Geometry check sheet. Reference: the model listing, model coordinates, mm. A direction names the side the tool comes from. Round coordinates to 2 decimals unless told otherwise and drop trailing zeros. Loops run counter-clockwise (first coordinate to the right, second up) from the corner with the lowest first, then second, coordinate; pieces in that order, holes last. Notation, with made-up numbers: (87, 44.25) - (113, 44.25) arc R30 cw to (113, 80.25) - close; hole circle Ø5 at (43.5, -24). An arc over 180 degrees is marked (long way). Answer in a Markdown table with one row per item. Add a question column.
Autodesk Inventor part; units mm, degrees
ref_plane "YZ Plane" through (0, 0, 0) normal (1, 0, 0) x (0, 1, 0)
ref_plane "XZ Plane" through (0, 0, 0) normal (0, 1, 0) x (-1, 0, 0)
ref_plane "XY Plane" through (0, 0, 0) normal (0, 0, 1) x (1, 0, 0)
sketch "Sketch1" plane through (0, 0, 0) normal (0, 1, 0) x (-1, 0, 0)
  line L0 (17.5, 17.5) -> (-17.5, 17.5)
  line L1 (-17.5, 17.5) -> (-17.5, -17.5)
  line L2 (-17.5, -17.5) -> (17.5, -17.5)
  line L3 (17.5, -17.5) -> (17.5, 17.5)
  line L4 (17.5, 17.5) -> (-17.5, -17.5) construction
  line L5 (-17.5, 17.5) -> (17.5, -17.5) construction
  point P0 (0, 0)
  dimension "d0" = 35
  dimension "d1" = 35
extrude "Extrusion1" add sketch "Sketch1" along normal blind 35
sketch "Sketch2" plane through (0, 35, 0) normal (0, 1, 0) x (1, 0, 0)
  line L0 (-2.3616, -50.7705) -> (15.6384, -50.7705)
  line L1 (15.6384, -50.7705) -> (15.6384, -44.7705)
  line L2 (15.6384, -44.7705) -> (-2.3616, -44.7705)
  line L3 (-2.3616, -44.7705) -> (-2.3616, -50.7705)
  line L4 (-2.3616, -50.7705) -> (15.6384, -44.7705) construction
  line L5 (15.6384, -50.7705) -> (-2.3616, -44.7705) construction
  circle A0 centre (6.6384, -47.7705) radius 11
  line L6 (-10.8616, -65.2705) -> (24.1384, -65.2705)
  line L7 (24.1384, -65.2705) -> (24.1384, -30.2705)
  line L8 (24.1384, -30.2705) -> (-10.8616, -30.2705)
  line L9 (-10.8616, -30.2705) -> (-10.8616, -65.2705)
  line L10 (-10.8616, -65.2705) -> (24.1384, -30.2705) construction
  line L11 (24.1384, -65.2705) -> (-10.8616, -30.2705) construction
  circle A1 centre (6.6384, -47.7705) radius 28.5
  circle A2 centre (0, 0) radius 10.5
  line L12 (-8.5, 2.75) -> (8.5, 2.75)
  line L13 (8.5, 2.75) -> (8.5, -2.75)
  line L14 (8.5, -2.75) -> (-8.5, -2.75)
  line L15 (-8.5, -2.75) -> (-8.5, 2.75)
  line L16 (-8.5, 2.75) -> (8.5, -2.75) construction
  line L17 (8.5, 2.75) -> (-8.5, -2.75) construction
  point P0 (-38.3616, 79.7295)
  dimension "d4" = 18
  dimension "d5" = 6
  dimension "d6" = 22
  dimension "d7" = 35
  dimension "d8" = 35
  dimension "d9" = 21
  dimension "d10" = 17
  dimension "d11" = 5.5
extrude "Extrusion2" cut sketch "Sketch2" against normal blind 22 contours L12 L13 L14 L15
extrude "Extrusion3" cut sketch "Sketch2" against normal blind 1.9 contours A2
sketch "Sketch3" plane through (-17.5, 0, 17.5) normal (0, 0, 1) x (1, 0, 0)
  line L0 (7, 35) -> (28, 35) construction
  line L1 (17.5, 35) -> (17.5, 22.6) construction
  point P0 (17.5, 0)
  dimension "d16" = 12.4
hole "Hole1" at (0, 22.6, 17.5) direction (0, 0, -1) diameter 6.5 end through all
sketch "Sketch4" plane through (0, 0, 0) normal (0, -1, 0) x (1, 0, 0)
  point P0 (0, 0)
hole "Hole2" at (0, 0, 0) direction (0, 1, 0) diameter 4.917 depth 11
sketch "Sketch6" plane through (0, 0, 0) normal (0, -1, 0) x (1, 0, 0)
  line L0 (-17.5, -17.5) -> (-17.5, 17.5) construction
  line L1 (17.5, 17.5) -> (-17.5, 17.5) construction
  line L2 (-17.5, 17.5) -> (-17.5, -17.5) construction
  line L3 (-17.5, -17.5) -> (17.5, -17.5) construction
  line L4 (17.5, -17.5) -> (17.5, 17.5) construction
  line L5 (17.5, 17.5) -> (-17.5, -17.5) construction
  line L6 (-17.5, 17.5) -> (17.5, -17.5) construction
  line L7 (9, -9) -> (-9, -9) construction
  line L8 (-9, -9) -> (-9, 9) construction
  line L9 (-9, 9) -> (9, 9) construction
  line L10 (9, 9) -> (9, -9) construction
  line L11 (9, -9) -> (-9, 9) construction
  line L12 (-9, -9) -> (9, 9) construction
  point P0 (0, 0)
  dimension "d63" = 18
  dimension "d64" = 18
hole "Hole3" at (9, 0, 9) at (-9, 0, -9) direction (0, 1, 0) diameter 5 depth 11
sketch "Sketch7" plane through (0, 35, 0) normal (0, 1, 0) x (1, 0, 0)
  line L0 (-8.5, 2.75) -> (8.5, 2.75) construction
  line L1 (8.5, 2.75) -> (17.5, 2.75) construction
  line L2 (17.5, -17.5) -> (17.5, 17.5) construction
  line L3 (8.5, 2.75) -> (8.5, -2.75)
  line L4 (17.5, 2.75) -> (8.5, 2.75)
  line L5 (8.5, 2.75) -> (8.5, -2.75)
  line L6 (8.5, -2.75) -> (17.5, -2.75)
  line L7 (17.5, -2.75) -> (17.5, 2.75)
  point P0 (0, 0)
extrude "Extrusion4" cut sketch "Sketch7" against normal up to surface (22 mm away)
sketch "Sketch8" plane through (0, 35, 0) normal (0, 1, 0) x (1, 0, 0)
  line L0 (17.5, 2.75) -> (-8.5, 2.75)
  line L1 (-8.5, 2.75) -> (-11, 2.75)
  line L2 (-11, 2.75) -> (-11, -2.75)
  line L3 (-11, -2.75) -> (-8.5, -2.75)
  line L4 (-8.5, -2.75) -> (-8.5, 2.75)
  line L5 (-8.5, 2.75) -> (-10.1335, 2.75) construction
  arc A0 (10.1335, 2.75) -> (10.1335, -2.75) centre (0, 0) ccw construction
  dimension "d44" = 2.5
  dimension "d45" = 1.6335
extrude "Extrusion5" cut sketch "Sketch8" against normal up to surface (22 mm away)
fillet "Fillet2" radius 2.5 2 edges at (-11, 24, 2.75) (-11, 24, -2.75)
properties part number "Holder"
Q1. Cross-section at D-D, the plane z = 12. Enter the section's corners in (x, y), plus the area to 3 significant figures.
Q2. Cross-section at B-B, the plane y = 4.5. Enter the section's corners in (x, z).
Q3. Scan lines: line 1 (X direction, y = 22.6, z = -12.75); line 2 (Z direction, x = 6, y = 16); line 3 (X direction, y = 7, z = 0). Record each from-to range of solid material in increasing order. Write a range as from..to.
Q4. Set-up check for faces 4 (the flat face through (4, 24, 2.75)), 5 (the cylindrical face through (-0.2, 34.1, -10.5)), 6 (the cylindrical face through (-0.738, 5.577, -2.345)), 7 (the cylindrical face through (-0.98, 19.5, -10.23)): record each of +Z, -Z, +X, -X, +Y, -Y from which the full face is reachable in a straight line by a thin tool's end or side.
Q5. Release check for a two-part mould opening along X. For faces 1 (the flat face through (-17.5, 17, 0)), 2 (the flat face through (0, 11, 0)), 3 (the cylindrical face through (-10.287, 23.846, -1.998)) record: +X half, -X half, draft (parallel to the pull), parting line (faces both ways), or undercut.
Q6. Depth check by flat-ended pin: P1, Ø0.6, axis at y = 26, z = 0, coming from the +X side; P2, Ø1.5, axis at x = -8, z = -9.5, coming from the -Y side; P3, Ø8, axis at x = 0, z = 0, coming from the +Y side; P4, Ø4, axis at x = 0, y = 22.6, coming from the -Z side. Enter the tip coordinate at first touch or a pass-through.
Q7. Cross-section at C-C, the plane y = 20. Enter the section's corners in (x, z).
Q8. Cross-section at A-A, the plane x = 0. Enter the section's corners in (y, z).
Check sheet entries:
| question | item | result |
|---|---|---|
| 1 | outline | (-17.5, 0) - (17.5, 0) - (17.5, 35) - (-17.5, 35) - close; hole circle Ø6.5 at (0, 22.6) |
| 1 | area | 1,190 mm² |
| 2 | outline | (-17.5, -17.5) - (17.5, -17.5) - (17.5, 17.5) - (-17.5, 17.5) - close; hole circle Ø5 at (-9, -9); hole circle Ø4.92 at (0, 0); hole circle Ø5 at (9, 9) |
| 3 | line 1 | -17.5..-3.25, 3.25..17.5 |
| 3 | line 2 | -17.5..-2.75, 2.75..17.5 |
| 3 | line 3 | -17.5..-2.46, 2.46..17.5 |
| 4 | face 4 | +X, +Y |
| 4 | face 5 | +Y |
| 4 | face 6 | -Y |
| 4 | face 7 | +Z, -Z |
| 5 | face 1 | -X half |
| 5 | face 2 | undercut |
| 5 | face 3 | +X half |
| 6 | P1 | x = -11 |
| 6 | P2 | y = 11 |
| 6 | P3 | y = 33.1 |
| 6 | P4 | through |
| 7 | outline | (-17.5, -17.5) - (-1.95, -17.5) - (-1.95, -2.75) - (-8.5, -2.75) arc R2.5 cw to (-11, -0.25) - (-11, 0.25) arc R2.5 cw to (-8.5, 2.75) - (-1.95, 2.75) - (-1.95, 17.5) - (-17.5, 17.5) - close; (1.95, -17.5) - (17.5, -17.5) - (17.5, -2.75) - (1.95, -2.75) - close; (1.95, 2.75) - (17.5, 2.75) - (17.5, 17.5) - (1.95, 17.5) - close |
| 8 | outline | (0, -17.5) - (19.35, -17.5) - (19.35, -2.75) - (13, -2.75) - (13, 2.75) - (19.35, 2.75) - (19.35, 17.5) - (0, 17.5) - (0, 2.46) - (11, 2.46) - (11, -2.46) - (0, -2.46) - close; (25.85, -17.5) - (35, -17.5) - (35, -10.5) - (33.1, -10.5) - (33.1, -2.75) - (25.85, -2.75) - close; (25.85, 2.75) - (33.1, 2.75) - (33.1, 10.5) - (35, 10.5) - (35, 17.5) - (25.85, 17.5) - close |
